```python
from build123d import *

# Parameters (mm, degrees)
F0_R     = 4
F0_R_2   = 12.5
F0_R_3   = 3.795856
F1_DEPTH = 10


with BuildPart() as f1:
    # F0 (on Top) → F1 (new body)
    with BuildSketch(Plane.XY):
        with BuildLine():
            ThreePointArc((100, 65), (97.071068, 72.071068), (90, 75))
            Line((90, 75), (-90, 75))
            ThreePointArc((-90, 75), (-97.071068, 72.071068), (-100, 65))
            Line((-100, 65), (-100, -65))
            ThreePointArc((-100, -65), (-97.071068, -72.071068), (-90, -75))
            Line((-90, -75), (90, -75))
            ThreePointArc((90, -75), (97.071068, -72.071068), (100, -65))
            Line((100, -65), (100, 65))
        make_face()
        with Locations((-90, -65)):
            Circle(F0_R, mode=Mode.SUBTRACT)
        with Locations((0, -65)):
            Circle(F0_R, mode=Mode.SUBTRACT)
        with Locations((90, -65)):
            Circle(F0_R, mode=Mode.SUBTRACT)
        with Locations((-75, 0)):
            Circle(F0_R_2, mode=Mode.SUBTRACT)
        with Locations((-90, 65)):
            Circle(F0_R, mode=Mode.SUBTRACT)
        Circle(F0_R_2, mode=Mode.SUBTRACT)
        with Locations((75, 0)):
            Circle(F0_R_2, mode=Mode.SUBTRACT)
        with Locations((0, 65)):
            Circle(F0_R_3, mode=Mode.SUBTRACT)
        with Locations((90, 65)):
            Circle(F0_R, mode=Mode.SUBTRACT)
    extrude(amount=F1_DEPTH)


solid = f1.part
```
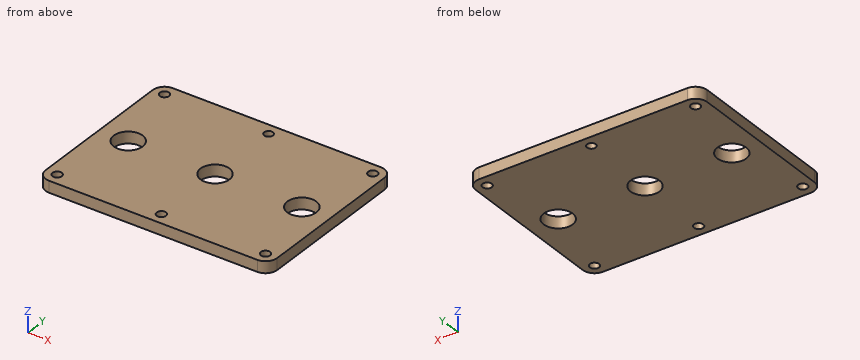
Geometry: final body of the model. Coordinates: model frame, mm. Round coordinates to 2 decimals unless told otherwise and drop trailing zeros. Loops run counter-clockwise (first coordinate to the right, second up) from the corner with the lowest first, then second, coordinate; pieces in that order, holes last. Notation, with made-up numbers: (68.25, 43) -> (98.25, 43) arc R21 cw to (98.25, 60) -> close; hole circle Ø7 at (5, 23). An arc over 180 degrees is marked (long way). Use one line per item in the form item = value. Start each with the question number.
1) Line query: L1, parallel to Y at x = -90, z = 8; L2, parallel to Y at x = 0, z = 2.5; L3, parallel to X at y = -7.5, z = 5. Output: solid intervals per line, ascending.
2) Section B-B on y = 0. Output: boundary loops of the cut face in (x, z), then the cut area to 3 significant figures.
3) Section D-D on x = 75. Output: boundary loops of the cut face in (y, z), then the cut area to 3 significant figures.
4) Section C-C on x = 0. Output: boundary loops of the cut face in (y, z).
5) Section A-A on z = 7. Give the number of separate pieces and of enclosed holes in the cut face, then the cut area to 3 significant figures.
Response:
q1.L1 = -75 to -69, -61 to 61, 69 to 75
q1.L2 = -75 to -69, -61 to -12.5, 12.5 to 61.2, 68.8 to 75
q1.L3 = -100 to -85, -65 to -10, 10 to 65, 85 to 100
q2.outline = (-100, 0) -> (-87.5, 0) -> (-87.5, 10) -> (-100, 10) -> close; (-62.5, 0) -> (-12.5, 0) -> (-12.5, 10) -> (-62.5, 10) -> close; (12.5, 0) -> (62.5, 0) -> (62.5, 10) -> (12.5, 10) -> close; (87.5, 0) -> (100, 0) -> (100, 10) -> (87.5, 10) -> close
q2.area = 1,250 mm^2
q3.outline = (-75, 0) -> (-12.5, 0) -> (-12.5, 10) -> (-75, 10) -> close; (12.5, 0) -> (75, 0) -> (75, 10) -> (12.5, 10) -> close
q3.area = 1,250 mm^2
q4.outline = (-75, 0) -> (-69, 0) -> (-69, 10) -> (-75, 10) -> close; (-61, 0) -> (-12.5, 0) -> (-12.5, 10) -> (-61, 10) -> close; (12.5, 0) -> (61.2, 0) -> (61.2, 10) -> (12.5, 10) -> close; (68.8, 0) -> (75, 0) -> (75, 10) -> (68.8, 10) -> close
q5.separate_pieces = 1
q5.enclosed_holes = 9
q5.area = 28,100 mm^2
